Verification items for the finished model (mm, model axes). A direction names the side the tool comes from. Coordinates: 2 decimals unless noted, no trailing zeros. Loops run counter-clockwise (first coordinate to the right, second up) from the corner with the lowest first, then second, coordinate; pieces in that order, holes last.
Q1. Sectioned sample at D-D (z = 9). Enter the section's corners in (x, y), then the cut area to 3 significant figures.
Q2. Mould release check, pull along Y, two halves, no side actions. Record for faces 1 (the face through (11.5, -11.4, 5.5)), 2 (the face through (0, -8.5, 8)), 3 (the face through (4.269, 6.723, 3.204)): +Y half, -Y half, draft (parallel to the pull), parting line (faces both ways), or undercut.
Q3. Go/stop test with flat-tipped pins: P1, Ø8, axis at x = 3.5, y = -17, coming from the +Z side; P2, Ø2.5, axis at y = -8, z = 8.5, coming from the -X side; P3, Ø5.5, axis at x = -5.66, y = -5.66, coming from the +Z side. Record where each tip stops, or that it passes through.
Q4. Sectioned sample at B-B (z = 2.5). Enter the section's corners in (x, y).
Q5. Material ranges on probe 1 along Y at (x, z) = (0, 2.5); probe 2 along Y at (x, z) = (6.25, 8.25); probe 3 along X at (y, z) = (3, 3.75), recorded low to high.
Q6. Sectioned sample at C-C (y = -20). Enter the section's corners in (x, z), then the cut area to 3 significant figures.
Q7. Access from +Z, -Z, +X, -X, +Y, -Y to the whole of each face (thin tool, end or side, straight path). Record for faces 4 (the face through (-2.277, -5.501, 8.226)), 5 (the face through (7.955, -3.728, 8.274)), 6 (the face through (4.3, -21, 3)), 7 (the face through (-11.43, -7.9, 7.78)), 8 (the face through (-12, -6, 4)).
Q8. Sectioned sample at A-A (x = 0). Enter the section's corners in (y, z).
```python
from build123d import *

# Parameters (mm, degrees)
F0_R        = 1.75
F0_R_2      = 5.5
F1_DEPTH    = 10
F2_SIZE2    = 8
F2_SIZE     = 2
F3_SIZE2    = 2
F3_SIZE     = 8
F5_W        = 20
F5_H        = 8
F6_DEPTH    = 15
F7_R        = 3
F8_DEPTH    = 3.5
F9_T1_DEPTH = 7.3998501729
F9_T3_DEPTH = 7.1931423334
F10_R       = 2
F11_SIZE    = 0.5
F12_SIZE    = 1
F13_R       = 3
F14_R       = 20
F15_SIZE    = 1
F17_ANGLE   = 45


# Not quite as in the source:
# - a fillet or chamfer that OpenCascade refuses, or shapes differently, is made with other operations: its cross-section is extruded or revolved along the edge and cut away or added


with BuildPart() as f1:
    # F0 (on Top) → F1 (new body)
    with BuildSketch(Plane.XY):
        with BuildLine():
            Line((-9.1923881554, -26.1629509039), (8.4852813742, -8.4852813742))
            ThreePointArc((8.4852813742, -8.4852813742), (8.4852813742, 8.4852813742), (-8.4852813742, 8.4852813742))
            Line((-8.4852813742, 8.4852813742), (-26.1629509039, -9.1923881554))
            Line((-26.1629509039, -9.1923881554), (-20.7182286888, -14.6371103706))
            Line((-20.7182286888, -14.6371103706), (-15.4149278299, -9.3338095117))
            ThreePointArc((-15.4149278299, -9.3338095117), (-9.3338095117, -9.3338095117), (-9.3338095117, -15.4149278299))
            Line((-9.3338095117, -15.4149278299), (-14.6371103706, -20.7182286888))
            Line((-14.6371103706, -20.7182286888), (-9.1923881554, -26.1629509039))
        make_face()
        with Locations((0, -8)):
            Circle(F0_R, mode=Mode.SUBTRACT)
        with Locations((-8, 0)):
            Circle(F0_R, mode=Mode.SUBTRACT)
        Circle(F0_R_2, mode=Mode.SUBTRACT)
        with Locations((8, 0)):
            Circle(F0_R, mode=Mode.SUBTRACT)
        with Locations((0, 8)):
            Circle(F0_R, mode=Mode.SUBTRACT)
    extrude(amount=F1_DEPTH)

    # F2
    f2_edges = [f1.edges().sort_by_distance(p)[0] for p in [
        (-26.162951, -9.192388, 5),
    ]]
    f2_side = f1.faces().sort_by_distance((-23.44059, -11.914749, 5))[0]
    chamfer(f2_edges, length=F2_SIZE, length2=F2_SIZE2, reference=f2_side)

    # F3
    f3_edges = [f1.edges().sort_by_distance(p)[0] for p in [
        (-9.192388, -26.162951, 5),
    ]]
    f3_side = f1.faces().sort_by_distance((-0.353553, -17.324116, 5))[0]
    chamfer(f3_edges, length=F3_SIZE, length2=F3_SIZE2, reference=f3_side)

    # F5 (on offset) → F6 (cut, symmetric)
    with BuildSketch(Plane(origin=(0.5303300859, -0.5303300859, 0), x_dir=(0.7071067812, 0.7071067812, 0), z_dir=(0.7071067812, -0.7071067812, 0))):
        with Locations((-18.5, 10)):
            Rectangle(F5_W, F5_H)
    extrude(amount=F6_DEPTH, both=True, mode=Mode.SUBTRACT)

    # F7 (on face) → F8 (cut)
    with BuildSketch(Plane.XY.offset(10)):
        with BuildLine():
            Line((-7.8890872965, -4.1317279836), (-5.8786796564, -2.1213203436))
            ThreePointArc((-5.8786796564, -2.1213203436), (-5.8786796564, 2.1213203436), (-10.1213203436, 2.1213203436))
            Line((-10.1213203436, 2.1213203436), (-12.1317279836, 0.1109127035))
            Line((-12.1317279836, 0.1109127035), (-7.8890872965, -4.1317279836))
        make_face()
        with BuildLine():
            Line((0.1109127035, -12.1317279836), (2.1213203436, -10.1213203436))
            ThreePointArc((2.1213203436, -10.1213203436), (2.1213203436, -5.8786796564), (-2.1213203436, -5.8786796564))
            Line((-2.1213203436, -5.8786796564), (-4.1317279836, -7.8890872965))
            Line((-4.1317279836, -7.8890872965), (0.1109127035, -12.1317279836))
        make_face()
        with Locations((8, 0)):
            Circle(F7_R)
        with Locations((0, 8)):
            Circle(F7_R)
    extrude(amount=-F8_DEPTH, mode=Mode.SUBTRACT)

    # F9: fillet of radius 1 on 8 edges, made by hand

    # F9_s2 → F9_t1 (cut)
    with BuildSketch(Plane.XY.offset(6.5)):
        with BuildLine():
            ThreePointArc((-6.3230487903, -2.5656894774), (-5.4874259536, -2.2810888302), (-4.7519509308, -2.7692891419))
            Line((-4.7519509308, -2.7692891419), (-4.665551823, -2.7189384302))
            ThreePointArc((-4.665551823, -2.7189384302), (-4.9962431034, -2.0487935111), (-5.23125, -1.3394116012))
            Line((-5.23125, -1.3394116012), (-5.4171875, -1.3187416691))
            ThreePointArc((-5.4171875, -1.3187416691), (-5.9493903346, -2.0506096654), (-6.3937594684, -2.4949787993))
            Line((-6.3937594684, -2.4949787993), (-6.3230487903, -2.5656894774))
        make_face()
        with BuildLine():
            ThreePointArc((-2.5656894774, -6.3230487903), (-2.2810888302, -5.4874259536), (-2.7692891419, -4.7519509308))
            Line((-2.7692891419, -4.7519509308), (-2.7189384302, -4.665551823))
            ThreePointArc((-2.7189384302, -4.665551823), (-2.0487935111, -4.9962431034), (-1.3394116012, -5.23125))
            Line((-1.3394116012, -5.23125), (-1.3187416691, -5.4171875))
            ThreePointArc((-1.3187416691, -5.4171875), (-2.0506096654, -5.9493903346), (-2.4949787993, -6.3937594684))
            Line((-2.4949787993, -6.3937594684), (-2.5656894774, -6.3230487903))
        make_face()
    extrude(amount=F9_T1_DEPTH, mode=Mode.SUBTRACT)

    # F9_s4 → F9_t3 (cut)
    with BuildSketch(Plane.XY.offset(6.5)):
        with BuildLine():
            ThreePointArc((-6.23046875, 2.4225521987), (-5.4322290759, 2.2520250497), (-4.7728365385, 2.7331358139))
            ThreePointArc((-4.7728365385, 2.7331358139), (-5.0966500462, 2.06740376), (-5.328125, 1.3642155198))
            ThreePointArc((-5.328125, 1.3642155198), (-5.717119911, 1.9463962852), (-6.23046875, 2.4225521987))
        make_face()
        with BuildLine():
            ThreePointArc((2.4225521987, -6.23046875), (2.2520250497, -5.4322290759), (2.7331358139, -4.7728365385))
            ThreePointArc((2.7331358139, -4.7728365385), (2.06740376, -5.0966500462), (1.3642155198, -5.328125))
            ThreePointArc((1.3642155198, -5.328125), (1.9463962852, -5.717119911), (2.4225521987, -6.23046875))
        make_face()
        with BuildLine():
            ThreePointArc((6.23046875, -2.4225521987), (5.4322290759, -2.2520250497), (4.7728365385, -2.7331358139))
            ThreePointArc((4.7728365385, -2.7331358139), (5.0966500462, -2.06740376), (5.328125, -1.3642155198))
            ThreePointArc((5.328125, -1.3642155198), (5.717119911, -1.9463962852), (6.23046875, -2.4225521987))
        make_face()
        with BuildLine():
            ThreePointArc((6.23046875, 2.4225521987), (5.4322290759, 2.2520250497), (4.7728365385, 2.7331358139))
            ThreePointArc((4.7728365385, 2.7331358139), (5.0966500462, 2.06740376), (5.328125, 1.3642155198))
            ThreePointArc((5.328125, 1.3642155198), (5.717119911, 1.9463962852), (6.23046875, 2.4225521987))
        make_face()
        with BuildLine():
            ThreePointArc((-2.4225521987, 6.23046875), (-2.2520250497, 5.4322290759), (-2.7331358139, 4.7728365385))
            ThreePointArc((-2.7331358139, 4.7728365385), (-2.06740376, 5.0966500462), (-1.3642155198, 5.328125))
            ThreePointArc((-1.3642155198, 5.328125), (-1.9463962852, 5.717119911), (-2.4225521987, 6.23046875))
        make_face()
        with BuildLine():
            ThreePointArc((2.4225521987, 6.23046875), (2.2520250497, 5.4322290759), (2.7331358139, 4.7728365385))
            ThreePointArc((2.7331358139, 4.7728365385), (2.06740376, 5.0966500462), (1.3642155198, 5.328125))
            ThreePointArc((1.3642155198, 5.328125), (1.9463962852, 5.717119911), (2.4225521987, 6.23046875))
        make_face()
    extrude(amount=F9_T3_DEPTH, mode=Mode.SUBTRACT)

    # F10
    f10_edges = [f1.edges().sort_by_distance(p)[0] for p in [
        (2.474874, -14.495689, 8),
        (-14.495689, 2.474874, 8),
    ]]
    fillet(f10_edges, radius=F10_R)

    # F11
    f11_edges = [f1.edges().sort_by_distance(p)[0] for p in [
        (0.585786, -12.606602, 10),
        (-12.606602, 0.585786, 10),
        (-6.010408, -6.010408, 10),
        (2.474874, -13.667262, 10),
        (-13.667262, 2.474874, 10),
        (6.187184, -10.783378, 10),
        (8.485281, 8.485281, 10),
        (-10.783378, 6.187184, 10),
    ]]
    chamfer(f11_edges, length=F11_SIZE)

    # F12
    f12_edges = [f1.edges().sort_by_distance(p)[0] for p in [
        (-20.718229, -14.63711, 3),
        (-14.63711, -20.718229, 3),
    ]]
    chamfer(f12_edges, length=F12_SIZE)

    # F13
    f13_edges = [f1.edges().sort_by_distance(p)[0] for p in [
        (-10.606602, -24.748737, 3),
        (-24.748737, -10.606602, 3),
    ]]
    fillet(f13_edges, radius=F13_R)

    # F14
    f14_edges = [f1.edges().sort_by_distance(p)[0] for p in [
        (-3.535534, -20.506097, 3),
        (-20.506097, -3.535534, 3),
    ]]
    fillet(f14_edges, radius=F14_R)

    # F15
    f15_edges = [f1.edges().sort_by_distance(p)[0] for p in [
        (-13.096441, -22.258898, 6),
        (-10.508108, -23.948663, 6),
        (-7.122424, -22.658231, 6),
        (-3.628449, -20.387093, 6),
        (0.340158, -16.630405, 6),
        (-22.258898, -13.096441, 6),
        (-23.948663, -10.508108, 6),
        (-22.658231, -7.122424, 6),
    ]]
    chamfer(f15_edges, length=F15_SIZE)


with BuildPart() as f1_1:
    # F17: moved
    add(f1.part.rotate(Axis((0, 0, 12.5), (0, 0, 1)), F17_ANGLE))


solid = f1_1.part
```
Geometry check:
1. outline: (-12, -6.5) arc R2 ccw to (-10, -8.5) - (-8.66, -8.5) - (-8.66, -5.66) arc R3 cw to (-6.12, -2.69) arc R1 ccw to (-5.31, -1.44) arc R5.5 cw to (-5.31, 1.44) arc R1 ccw to (-6.12, 2.69) arc R3 cw (long way) to (-2.69, 6.12) arc R1 ccw to (-1.44, 5.31) arc R5.5 cw to (1.44, 5.31) arc R1 ccw to (2.69, 6.12) arc R3 cw (long way) to (6.12, 2.69) arc R1 ccw to (5.31, 1.44) arc R5.5 cw to (5.31, -1.44) arc R1 ccw to (6.12, -2.69) arc R3 cw to (8.66, -5.66) - (8.66, -8.5) - (10, -8.5) arc R2 ccw to (12, -6.5) - (12, 0) arc R12 ccw to (-12, 0) - close; (-2.66, -8.5) - (2.66, -8.5) - (2.66, -6.29) arc R1 ccw to (1.4, -5.32) arc R5.5 cw to (-1.4, -5.32) arc R1 ccw to (-2.66, -6.29) - close
1. area: 215 mm2
2. face 1: draft
2. face 2: -Y half
2. face 3: undercut
3. P1: stops at z = 6
3. P2: stops at x = -11.98
3. P3: stops at z = 6.5
4. outline: (-12, -14.54) arc R20 ccw to (-11.4, -19.39) - (-10.57, -22.73) arc R3 ccw to (-7.66, -25) - (-5.3, -25) - (-4.3, -24) - (-4.3, -17.5) arc R4.3 cw to (4.3, -17.5) - (4.3, -24) - (5.3, -25) - (7.66, -25) arc R3 ccw to (10.57, -22.73) - (11.4, -19.39) arc R20 ccw to (12, -14.54) - (12, 0) arc R12 ccw to (-12, 0) - close; hole circle Ø3.5 at (-5.66, -5.66); hole circle Ø3.5 at (-5.66, 5.66); hole circle Ø11 at (0, 0); hole circle Ø3.5 at (5.66, -5.66); hole circle Ø3.5 at (5.66, 5.66)
5. probe 1: y = -13.2 to -5.5, 5.5 to 12
5. probe 2: y = -2.72 to 2.72, 8.6 to 10.24
5. probe 3: x = -11.62 to -4.61, 4.61 to 11.62
6. outline: (-11.25, 0) - (-4.3, 0) - (-4.3, 6) - (-10.22, 6) - (-11.25, 5) - close; (4.3, 0) - (11.25, 0) - (11.25, 5) - (10.22, 6) - (4.3, 6) - close
6. area: 82.4 mm2
7. face 4: +Z
7. face 5: +Z, -Y
7. face 6: +Z, -Z, -Y
7. face 7: +Z, -X, -Y
7. face 8: +Z, -Z, -X, +Y, -Y
8. outline: (-13.2, 0) - (-5.5, 0) - (-5.5, 10) - (-8, 10) - (-8.5, 9.5) - (-8.5, 6) - (-13.2, 6) - close; (5.5, 0) - (12, 0) - (12, 9.5) - (11.5, 10) - (5.5, 10) - close
